Geometry: final body of the model. Coordinates: model frame, mm. Give positions to 0.01 mm unless a question says otherwise; leave off trailing zeros. Write each loop counter-clockwise with the first axis right and the second up, starting at its lowest first coordinate (ties: lowest second). Pieces come first, ordered by that corner, then holes.
Q1. Mould query, pull axis Y, two halves, no side actions, for faces 1 (the flat face through (-1, 1, 3)), 2 (the cylindrical face through (-26.255, -20.988, 1.521)), 3 (the cylindrical face through (-13.516, -27.145, 1.521)). Classes: +Y half, -Y half, draft (parallel to the pull), parting line (faces both ways), or undercut.
Q2. Pin query (flat end, axial travel): pin 1 Ø4.5 at (x, y) = (-31.5, -28.67) entering from -Z; pin 2 Ø0.9 at (x, z) = (101.5, 1.5) entering from +Y; pin 3 Ø0.9 at (x, z) = (101.5, 1.5) entering from -Y. Return the tip coordinate at first contact, or that it passes through.
Q3. Section D-D (z = 1.15). State how many separate pieces and enclosed holes the cut face has, plus the area to 3 significant figures.
Q4. Section B-B (y = -36). Return the cut outline in (x, z), plus the area to 3 significant figures.
Q5. Line query: line 1 (X direction, y = -45, z = 1.55); line 2 (Y direction, x = 2, z = 2.1); line 3 (Y direction, x = -23.5, z = 1.7). Output: solid intervals per line, ascending.
Q6. Section C-C (x = -23.5). Return the cut outline in (y, z).
Q7. Section A-A (x = 89). Return the cut outline in (y, z).
Autodesk Fusion 360 part; units mm, degrees
sketch "Esquisse1" plane through (0, 0, 0) normal (0, 0, 1) x (1, 0, 0)
  line L0 (103, -50) -> (-103, -50)
  line L1 (-103, -50) -> (-103, 50)
  line L2 (-103, 50) -> (103, 50)
  line L3 (103, 50) -> (103, -50)
  line L4 (103, -50) -> (-103, 50) construction
  line L5 (-103, -50) -> (103, 50) construction
  line L6 (-100, -53) -> (100, -53)
  line L7 (100, -53) -> (100, 53)
  line L8 (100, 53) -> (-100, 53)
  line L9 (-100, 53) -> (-100, -53)
  line L10 (-100, -53) -> (100, 53) construction
  line L11 (100, -53) -> (-100, 53) construction
  dimension "d1" = 206
  dimension "d2" = 100
  dimension "d41" = 200
  dimension "d42" = 106
extrude "Extrusion1" add sketch "Esquisse1" along normal blind 3
sketch "Esquisse3" plane through (0, 0, 3) normal (0, 0, 1) x (-1, 0, 0)
  line L0 (100, -50) -> (103, -50)
  line L1 (103, -50) -> (103, 50)
  line L2 (103, 50) -> (100, 50)
  line L3 (-103, 50) -> (-103, -50)
  line L4 (-4.6, -3.6) -> (-92.4, -3.6)
  line L5 (-92.4, -3.6) -> (-92.4, 38.6)
  line L6 (-92.4, 38.6) -> (-4.6, 38.6)
  line L7 (-4.6, 38.6) -> (-4.6, -3.6)
  line L8 (-4.6, -3.6) -> (-92.4, 38.6) construction
  line L9 (-92.4, -3.6) -> (-4.6, 38.6) construction
  line L10 (-2, -10) -> (-95, -10)
  line L11 (-95, -10) -> (-95, 45)
  line L12 (-95, 45) -> (-2, 45)
  line L13 (-2, 45) -> (-2, -10)
  line L14 (-2, -10) -> (-95, 45) construction
  line L15 (-95, -10) -> (-2, 45) construction
  line L16 (103, 50) -> (103, -50)
  line L17 (-100, -50) -> (-100, -53)
  line L18 (-100, -53) -> (100, -53)
  line L19 (100, -53) -> (100, -50)
  line L20 (100, 50) -> (100, 53)
  line L21 (100, 53) -> (-100, 53)
  line L22 (-100, 53) -> (-100, 50)
  line L23 (-100, 50) -> (-103, 50)
  line L24 (-103, -50) -> (-100, -50)
  circle A0 centre (-2, 45) radius 1.5
  circle A1 centre (-95, 45) radius 1.5
  circle A2 centre (-95, -10) radius 1.5
  circle A3 centre (-2, -10) radius 1.5
  line L25 (15.5, 40.6667) -> (31.5, 40.6667)
  line L26 (35.5, 36.6667) -> (35.5, 12.6667)
  line L27 (31.5, 8.6667) -> (15.5, 8.6667)
  line L28 (11.5, 12.6667) -> (11.5, 36.6667)
  line L29 (11.5, 40.6667) -> (35.5, 8.6667) construction
  line L30 (35.5, 40.6667) -> (11.5, 8.6667) construction
  circle A4 centre (31.5, 28.6667) radius 2.5
  circle A5 centre (15.5, 28.6667) radius 2.5
  arc A6 (31.5, 8.6667) -> (35.5, 12.6667) centre (31.5, 12.6667) ccw
  arc A7 (11.5, 12.6667) -> (15.5, 8.6667) centre (15.5, 12.6667) ccw
  arc A8 (15.5, 40.6667) -> (11.5, 36.6667) centre (15.5, 36.6667) ccw
  arc A9 (35.5, 36.6667) -> (31.5, 40.6667) centre (31.5, 36.6667) ccw
  circle A10 centre (23.5, 16.6667) radius 5.125
  line L31 (100, 53) -> (-100, 53)
  line L32 (14, -6) -> (86, -6)
  line L33 (86, -6) -> (86, -44)
  line L34 (86, -44) -> (14, -44)
  line L35 (14, -44) -> (14, -6)
  line L36 (14, -6) -> (86, -44) construction
  line L37 (86, -6) -> (14, -44) construction
  line L38 (-92.4, 30.15) -> (-96.1, 30.15)
  line L39 (-96.1, 30.15) -> (-96.1, 4.85)
  line L40 (-96.1, 4.85) -> (-92.4, 4.85)
  line L41 (-92.4, 4.85) -> (-92.4, 30.15)
  line L42 (-92.4, 30.15) -> (-96.1, 4.85) construction
  line L43 (-96.1, 30.15) -> (-92.4, 4.85) construction
  line L44 (-92.4, 4.85) -> (-96.1, 7.8397)
  line L45 (-92.4, 30.15) -> (-96.1, 27.8397)
  line L46 (14, -19) -> (12, -19)
  line L47 (12, -19) -> (12, -31)
  line L48 (12, -31) -> (14, -31)
  line L49 (14, -31) -> (14, -19)
  line L50 (14, -19) -> (12, -31) construction
  line L51 (12, -19) -> (14, -31) construction
  line L52 (50, -25) -> (50, -44)
  line L53 (86, -19) -> (88, -19)
  line L54 (86, -31) -> (86, -19)
  line L55 (88, -31) -> (86, -31)
  line L56 (88, -19) -> (86, -31) construction
  line L57 (88, -19) -> (88, -31)
  line L58 (86, -19) -> (88, -31) construction
  point P0 (-48.5, 17.5)
  point P1 (-48.5, 17.5)
  point P2 (23.5, 24.6667)
  point P3 (50, -25)
  point P4 (-94.25, 17.5)
  point P5 (13, -25)
  point P6 (87, -25)
  dimension "d26" = 3
  dimension "d27" = 100
  dimension "d30" = 87.8
  dimension "d31" = 42.2
  dimension "d34" = 93
  dimension "d35" = 55
  dimension "d44" = 3
  dimension "d45" = 3
  dimension "d46" = 3
  dimension "d47" = 3
  dimension "d48" = 24
  dimension "d49" = 32
  dimension "d50" = 5
  dimension "d51" = 12
  dimension "d52" = 4
  dimension "d53" = 5
  dimension "d54" = 12
  dimension "d55" = 4
  dimension "d56" = 4
  dimension "d57" = 4
  dimension "d58" = 4
  dimension "d59" = 4
  dimension "d60" = 10.25
  dimension "d61" = 8
  dimension "d62" = 12
  dimension "d63" = 8
  dimension "d64" = 8
  dimension "d65" = 72
  dimension "d66" = 38
  dimension "d67" = 53
  dimension "d68" = 200
  dimension "d69" = 79.5
  dimension "d70" = 28
  dimension "d71" = 36.3333
  dimension "d72" = 25.3
  dimension "d73" = 3.7
  dimension "d74" = 21.1
  dimension "d75" = 20
  dimension "d76" = 12
  dimension "d77" = 2
  dimension "d78" = 19
extrude "Extrusion3" cut sketch "Esquisse3" against normal blind 3 contours L4 L5 L6 L7 L41 | L5 L11 L41 L44 L45 | L11 L39 L44 L45 | L10 L11 A2 | L10 L11 A2 | L11 L12 A1 | L11 L12 A1 | L10 L13 A3 | L10 L13 A3 | L12 L13 A0 | L12 L13 A0 | A4 | A5 | A10 | L32 L33 L34 L35 L49 L54 | L35 L46 L47 L48 L49 | L33 L53 L54 L55 L57
equation "d30 = 87.3 mm + 0.5 mm"
equation "d31 = 41.7 mm + 0.5 mm"
equation "d52 = ( d48 - 16 mm ) / 2"
equation "d54 = d51"
equation "d55 = d52"
equation "d57 = d56"
equation "d58 = d57"
equation "d59 = d56"
equation "d62 = d48 / 2"
equation "d67 = d68 / 4 + 3 mm"
equation "d69 = d67 * 3 / 2"
equation "d70 = d27 / 4 + 3 mm"
equation "d71 = d27 / 3 + 3 mm"
equation "d74 = d31 / 2"
equation "d78 = d66 / 2"
Computed:
1. face 1: draft
1. face 2: undercut
1. face 3: undercut
2. pin 1: passes through
2. pin 2: stops at y = 50
2. pin 3: stops at y = -50
3. separate pieces: 1
3. enclosed holes: 9
3. area: 15,100 mm2
4. outline: (-103, 0) - (4.6, 0) - (4.6, 3) - (-103, 3) - close; (92.4, 0) - (103, 0) - (103, 3) - (92.4, 3) - close
4. area: 355 mm2
5. line 1: x = -103 to 0.5, 3.5 to 93.5, 96.5 to 103
5. line 2: y = -53 to -46.5, -43.5 to 8.5, 11.5 to 53
5. line 3: y = -53 to -21.79, -11.54 to 6, 44 to 53
6. outline: (-53, 0) - (-21.79, 0) - (-21.79, 3) - (-53, 3) - close; (-11.54, 0) - (6, 0) - (6, 3) - (-11.54, 3) - close; (44, 0) - (53, 0) - (53, 3) - (44, 3) - close
7. outline: (-53, 0) - (-38.6, 0) - (-38.6, 3) - (-53, 3) - close; (3.6, 0) - (53, 0) - (53, 3) - (3.6, 3) - close
